Verification items for the finished model (mm, model axes). Face numbers are marked on the shaded views. Coordinates: 2 decimals unless noted, no trailing zeros. Order: outer loops, then holes, each group sorted by start corner. A loop starts at its lowest first (then second) coordinate and runs counter-clockwise, first axis right, second up. Notation, with made-up numbers: M 27,51.25 L 34,51.25 A14 ccw 34,73.25 Z; hole C 52.5,-13.75 d2. An arc over 180 degrees is marked long. Return JSON: item names as keys, results as strings.
```python
from build123d import *

# Parameters (mm, degrees)
SKETCH_1_R                      = 12.5
EXTRUDE_1_DEPTH                 = 8
SKETCH_2_R                      = 3.2
CUT_EXTRUDE_1_DEPTH             = 6
CUT_EXTRUDE_2_REACH             = 21.404
SKETCH_3_R                      = 1
CUT_EXTRUDE_2_DIRECTION_2_REACH = 21.404


with BuildPart() as part:
    # 草图1 → 凸台-拉伸1 (new body)
    with BuildSketch(Plane(origin=(0, 0, 0), x_dir=(0, 0, -1), z_dir=(1, 0, 0))):
        Circle(SKETCH_1_R)
    extrude(amount=EXTRUDE_1_DEPTH)

    # 草图2 → 切除-拉伸1 (cut)
    with BuildSketch(Plane.ZY):
        Circle(SKETCH_2_R)
    extrude(amount=-CUT_EXTRUDE_1_DEPTH, mode=Mode.SUBTRACT)

    # 草图3 → 切除-拉伸2 (cut, up to next)
    with BuildSketch(Plane(origin=(0, 0, 0), x_dir=(1, 0, 0), z_dir=(0, 1, 0)), mode=Mode.PRIVATE) as cut_extrude_2_sk1:
        with Locations(Location((3, 0, 0), (0, 0, 270))):
            Circle(SKETCH_3_R)
    cut_extrude_2_tool1 = extrude(cut_extrude_2_sk1.sketch, amount=-CUT_EXTRUDE_2_REACH, mode=Mode.PRIVATE) & part.part
    add(cut_extrude_2_tool1.solids().sort_by_distance((3, 0, 0))[0], mode=Mode.SUBTRACT)

    # 草图3 → 切除-拉伸2 direction 2 (cut, up to next)
    with BuildSketch(Plane(origin=(0, 0, 0), x_dir=(1, 0, 0), z_dir=(0, 1, 0)), mode=Mode.PRIVATE) as cut_extrude_2_direction_2_sk1:
        with Locations(Location((3, 0, 0), (0, 0, 270))):
            Circle(SKETCH_3_R)
    cut_extrude_2_direction_2_tool1 = extrude(cut_extrude_2_direction_2_sk1.sketch, amount=CUT_EXTRUDE_2_DIRECTION_2_REACH, mode=Mode.PRIVATE) & part.part
    add(cut_extrude_2_direction_2_tool1.solids().sort_by_distance((3, 0, 0))[0], mode=Mode.SUBTRACT)


solid = part.part
```
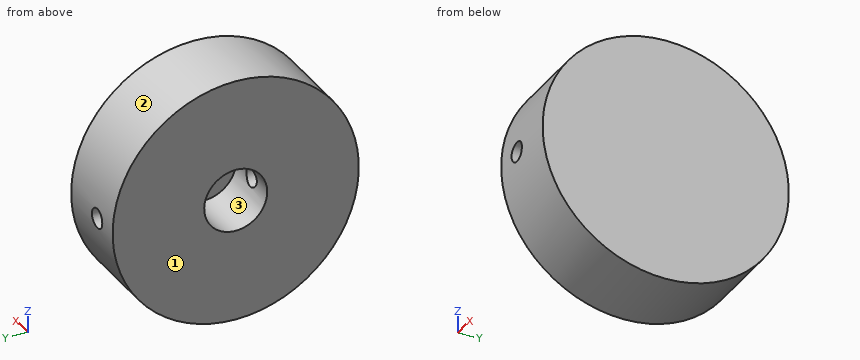
Q1. Cross-section at A-A, the plane z = 0. Record the boundary of the cut face in (x, y), and give its area (3 significant figures).
Values:
{"outline": "M 0,-12.5 L 2,-12.5 L 2,-3.2 L 0,-3.2 Z; M 0,3.2 L 2,3.2 L 2,12.5 L 0,12.5 Z; M 4,-12.5 L 8,-12.5 L 8,12.5 L 4,12.5 L 4,3.2 L 6,3.2 L 6,-3.2 L 4,-3.2 Z", "area": "124 mm^2"}
Q2. Cross-section at D-D, the plane x = 1.5. Record the boundary of the cut face in (y, z), and give its area (3 significant figures).
Values:
{"outline": "C 0,0 d25; hole C 0,0 d6.4", "area": "459 mm^2"}
Q3. Cross-section at B-B, the plane y = 0. Record the boundary of the cut face in (x, z), and give its area (3 significant figures).
Values:
{"outline": "M 0,-12.5 L 8,-12.5 L 8,12.5 L 0,12.5 L 0,3.2 L 6,3.2 L 6,-3.2 L 0,-3.2 Z", "area": "162 mm^2"}
Q4. Cross-section at C-C, the plane x = 3. Record the boundary of the cut face in (y, z), and give its area (3 significant figures).
Values:
{"outline": "M -12.46,-1 A12.5 ccw 12.46,-1 L 3.04,-1 A3.2 cw -3.04,-1 Z; M -12.46,1 L -3.04,1 A3.2 cw 3.04,1 L 12.46,1 A12.5 ccw Z", "area": "421 mm^2"}
Q5. Draft check along Y on the marked faces 1, 2 and 3. Enter one of: pulls with the +Y half, pulls with the -Y half, needs draft (parallel to the pull), parting line crosses it, or undercut.
Values:
{"face 1": "needs draft", "face 2": "parting line crosses it", "face 3": "undercut"}
Q6. Go/stop test with flat-tipped pins: pin 1 (1.9 mm diameter, centred on y = -0.5, z = 1, fed in from -X); pin 2 (1.6 mm diameter, centred on x = 3, z = 0, fed in from +Y); pin 3 (1 mm diameter, centred on x = 2.5, y = 3, fed in from -Z). Record where each tip stops, or that it passes through.
Values:
{"pin 1": "x = 6", "pin 2": "through", "pin 3": "z = -12.25"}
Q7. Material ranges on line 1 along X through (y, z) = (-10, 0); line 2 along X through (y, z) = (-0.5, 2.25); line 3 along Z through (x, y) = (3, 7.5), recorded low to high.
Values:
{"line 1": "0 to 2, 4 to 8", "line 2": "6 to 8", "line 3": "-10 to -1, 1 to 10"}
